from build123d import *

# Parameters (mm, degrees)
CROQUIS1_W              = 20
CROQUIS1_H              = 10
SALIENTE_EXTRUIR1_DEPTH = 2
CROQUIS2_W              = 10
CROQUIS2_H              = 10
CROQUIS2_R              = 2.6
SALIENTE_EXTRUIR2_DEPTH = 10
REDONDEO1_R             = 5


with BuildPart() as part:
    # Croquis1 → Saliente-Extruir1 (new body)
    with BuildSketch(Plane(origin=(0, 0, 0), x_dir=(1, 0, 0), z_dir=(0, 1, 0))):
        with Locations((10, 5)):
            Rectangle(CROQUIS1_W, CROQUIS1_H)
    extrude(amount=SALIENTE_EXTRUIR1_DEPTH)

    # Croquis2 → Saliente-Extruir2 (add)
    with BuildSketch(Plane.XY):
        with Locations((10, 7)):
            Rectangle(CROQUIS2_W, CROQUIS2_H)
        with Locations((10, 7)):
            Circle(CROQUIS2_R, mode=Mode.SUBTRACT)
    extrude(amount=-SALIENTE_EXTRUIR2_DEPTH)

    # Redondeo1
    redondeo1_edges = [part.edges().sort_by_distance(p)[0] for p in [
        (15, 12, -5),
        (5, 12, -5),
    ]]
    fillet(redondeo1_edges, radius=REDONDEO1_R - 0.0001)  # a hair under: the kernel refuses the full size


solid = part.part
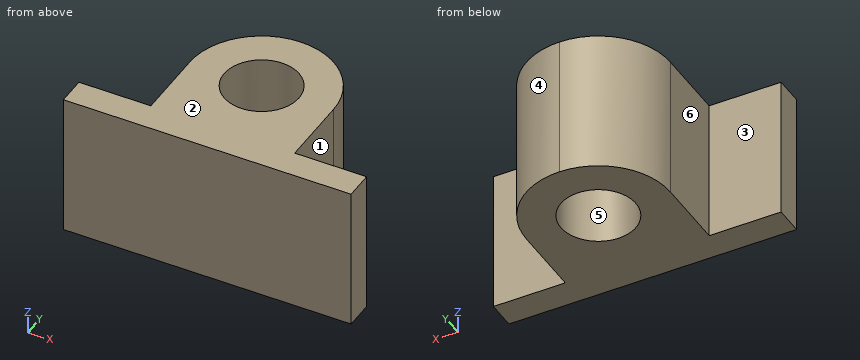
For this review, take the finished solid that the model builds, in its own axes (mm). Face numbers are marked on the shaded views. A direction names the side the tool comes from. Give positions to 0.01 mm unless a question says otherwise; leave off trailing zeros. Order: outer loops, then holes, each group sorted by start corner. A loop starts at its lowest first (then second) coordinate and runs counter-clockwise, first axis right, second up. Notation, with made-up numbers: (27.5, -13) - (49.5, -13) arc R12 cw to (49.5, -1) - close; hole circle Ø10 at (63.5, 88.25). An arc over 180 degrees is marked (long way). Answer as a JSON object with one key per item and string values. Group by question number.
Item 1: Take a section at A-A on y = 6. Give the boundary of the cut face in (x, z), and give its area (3 significant figures).
Item 2: Take a section at D-D on x = 15.5. Give the boundary of the cut face in (y, z).
Item 3: Draft analysis for pull direction Y (two halves, no side actions). For the marked faces 4, 5 and 6, state which applies: pulls with the +Y half, pulls with the -Y half, needs draft (parallel to the pull), parting line crosses it, or undercut.
Item 4: Take a section at C-C on x = 8.5. Give the boundary of the cut face in (y, z), and give its area (3 significant figures).
Item 5: Wall thickness on line 1 along Y through (x, z) = (10, -7); line 2 along Y through (x, z) = (7.75, -7.5); line 3 along X through (y, z) = (8.5, -6): over which ranges is each line inside the solid? List them lowest first.
Item 6: Clearance check with flat-ended pins moving along their axes: pin 1 Ø4 at (x, y) = (10, 7) entering from -Z; pin 2 Ø1.5 at (y, z) = (3.5, -3) entering from +X; pin 3 Ø1.5 at (y, z) = (10.5, -4) entering from +X; pin 4 Ø4 at (y, z) = (5.5, -6) entering from -X. State where each tip first meets the part, or that it passes through.
Item 7: Machinability: for the marked faces 1, 2 and 3, which of the approach directions +Z, -Z, +X, -X, +Y, -Y give a long, thin tool a straight path to every point of the face, cutting with its end or side? Answer none if there is none.
Reported:
{
 "1": {"outline": "(5, -10) - (7.6, -10) - (7.6, 0) - (5, 0) - close; (12.4, -10) - (15, -10) - (15, 0) - (12.4, 0) - close", "area": "52.0 mm^2"},
 "2": {"outline": "(0, -10) - (2, -10) - (2, 0) - (0, 0) - close"},
 "3": {"face 4": "pulls with the +Y half", "face 5": "undercut", "face 6": "needs draft"},
 "4": {"outline": "(0, -10) - (4.88, -10) - (4.88, 0) - (0, 0) - close; (9.12, -10) - (11.77, -10) - (11.77, 0) - (9.12, 0) - close", "area": "75.2 mm^2"},
 "5": {"line 1": "0 to 4.4, 9.6 to 12", "line 2": "0 to 5.7, 8.3 to 11.47", "line 3": "5.23 to 7.88, 12.12 to 14.77"},
 "6": {"pin 1": "through", "pin 2": "x = 15", "pin 3": "x = 14.18", "pin 4": "x = 5"},
 "7": {"face 1": "+Z, -Z, +X, +Y", "face 2": "+Z, +X, -X, +Y, -Y", "face 3": "+Z, -Z, -X, +Y"}
}
